Autodesk Inventor part; units mm, degrees
ref_plane "YZ Plane" through (0, 0, 0) normal (1, 0, 0) x (0, 1, 0)
ref_plane "XZ Plane" through (0, 0, 0) normal (0, 1, 0) x (-1, 0, 0)
ref_plane "XY Plane" through (0, 0, 0) normal (0, 0, 1) x (1, 0, 0)
sketch "Szkic1" plane through (0, 0, 0) normal (0, 1, 0) x (-1, 0, 0)
  line L0 (0, 0) -> (0, -40)
  line L1 (0, 0) -> (44, 0)
  line L2 (44, 0) -> (44, -40)
  line L3 (0, -40) -> (44, -40)
  dimension "d0" = 40
  dimension "d1" = 44
extrude "Wyciągnięcie proste1" add sketch "Szkic1" along normal blind 3
sketch "Szkic2" plane through (0, 3, 0) normal (0, 1, 0) x (1, 0, 0)
  line L0 (0, 0) -> (0, 40)
  line L1 (0, 40) -> (-44, 40)
  line L2 (-44, 40) -> (-44, 0)
  line L3 (-44, 0) -> (0, 0)
  line L4 (-42, 2) -> (-42, 38)
  line L5 (-42, 38) -> (-2, 38)
  line L6 (-2, 38) -> (-2, 2)
  line L7 (-2, 2) -> (-42, 2)
  line L8 (-42, 38) -> (-42, 40)
  line L9 (-2, 38) -> (-2, 40)
  line L10 (-2, 2) -> (-2, 0)
  line L11 (-42, 2) -> (-42, 0)
  dimension "d4" = 2
extrude "Wyciągnięcie proste2" add sketch "Szkic2" along normal blind 10 contours L3 L10 L6 L9 L1 L0 | L3 L2 L1 L8 L4 L11
sketch "Szkic3" plane through (0, 0, 0) normal (0, -1, 0) x (1, 0, 0)
  line L0 (0, 0) -> (0, -40)
  line L1 (-44, 0) -> (0, 0)
  line L2 (-44, -40) -> (-44, 0)
  line L3 (0, -40) -> (-44, -40)
  line L4 (0, -20) -> (5, -20)
  line L5 (-44, -20) -> (-49, -20) construction
  line L6 (-49, -20) -> (-49, -22.5)
  line L7 (-49, -20) -> (-49, -17.5)
  line L8 (5, -20) -> (5, -22.5)
  line L9 (5, -22.5) -> (5, -20)
  line L10 (5, -20) -> (5, -17.5)
  line L11 (5, -17.5) -> (0, -17.5)
  line L12 (5, -22.5) -> (0, -22.5)
  line L13 (-49, -22.5) -> (-44, -22.5)
  line L14 (-49, -17.5) -> (-44, -17.5)
  dimension "d7" = 5
  dimension "d8" = 5
  dimension "d9" = 2.5
  dimension "d10" = 2.5
  dimension "d11" = 2.5
  dimension "d12" = 2.5
extrude "Wyciągnięcie proste3" add sketch "Szkic3" against normal blind 3 contours L11 L10 L4 L0 | L4 L8 L12 L0 | L2 L13 L6 L7 L14
sketch "Szkic4" plane through (0, 3, 0) normal (0, 1, 0) x (1, 0, 0)
  line L0 (5, 17.5) -> (5, 22.5)
  line L1 (5, 22.5) -> (0, 22.5)
  line L2 (0, 17.5) -> (0, 22.5)
  line L3 (0, 17.5) -> (5, 17.5)
  line L4 (5, 17.5) -> (4, 17.5)
  line L5 (4, 17.5) -> (4, 22.5)
  line L6 (4, 22.5) -> (5, 22.5)
  line L7 (5, 22.5) -> (5, 17.5)
  line L8 (-49, 22.5) -> (-49, 17.5)
  line L9 (-49, 17.5) -> (-44, 17.5)
  line L10 (-44, 22.5) -> (-44, 17.5)
  line L11 (-44, 22.5) -> (-49, 22.5)
  line L12 (-49, 17.5) -> (-48, 17.5)
  line L13 (-48, 17.5) -> (-48, 22.5)
  line L14 (-48, 22.5) -> (-49, 22.5)
  line L15 (-49, 22.5) -> (-49, 17.5)
  point P0 (0, 0)
  dimension "d15" = 1
  dimension "d16" = 1
extrude "Wyciągnięcie proste4" add sketch "Szkic4" along normal blind 4 contours L3 L5 L1 L0 | L11 L13 L9 L8
sketch "Szkic5" plane through (4, 3, -22.5) normal (-1, 0, 0) x (0, 0, 1)
  line L0 (5, 0) -> (0, 0)
  line L1 (5, 0) -> (5, 4)
  line L2 (0, 4) -> (5, 4)
  line L3 (0, 0) -> (0, 4)
  line L4 (5, 4) -> (0, 4)
  line L5 (0, 4) -> (0, 3)
  line L6 (0, 3) -> (5, 3)
  line L7 (5, 3) -> (5, 4)
  point P0 (22.5, -3)
  dimension "d19" = 5
  dimension "d20" = 1
extrude "Wyciągnięcie proste5" add sketch "Szkic5" along normal blind 1 contours L6 L3 L2 L1
sketch "Szkic6" plane through (-48, 3, -17.5) normal (1, 0, 0) x (0, 0, -1)
  line L0 (5, 0) -> (0, 0)
  line L1 (5, 0) -> (5, 4)
  line L2 (0, 4) -> (5, 4)
  line L3 (0, 0) -> (0, 4)
  line L4 (0, 4) -> (5, 4)
  line L5 (5, 4) -> (5, 3)
  line L6 (5, 3) -> (0, 3)
  line L7 (0, 3) -> (0, 4)
  point P0 (-17.5, -3)
  point P1 (0, 3)
  point P2 (5, 3)
  dimension "d23" = 5
  dimension "d24" = 1
extrude "Wyciągnięcie proste6" add sketch "Szkic6" along normal blind 1 contours L6 L3 L2 L1
fillet "Zaokrąglenie1" radius 0.3 18 edges at (-49, 0, -20) (5, 0, -20) (5, 7, -20) (-49, 7, -20) (-44, 0, -31.25) (0, 0, -31.25) (0, 0, -8.75) (2.5, 0, -17.5) (2.5, 0, -22.5) (-44, 0, -8.75) (-46.5, 0, -17.5) (-46.5, 0, -22.5) (0, 13, -20) (-44, 13, -20) (-47, 7, -20) (3, 7, -20) (3, 6, -20) (-47, 6, -20)
sketch "Szkic8" plane through (-42, 3, 0) normal (0, 0, 1) x (1, 0, 0)
  arc A0 (-1.7, 10) -> (-2, 9.7) centre (-1.7, 9.7) ccw
  line L0 (-2, -2.7) -> (-2, 9.7)
  arc A1 (-2, -2.7) -> (-1.7, -3) centre (-1.7, -2.7) ccw
  line L1 (-1.7, -3) -> (41.7, -3)
  arc A2 (41.7, -3) -> (42, -2.7) centre (41.7, -2.7) ccw
  line L2 (42, -2.7) -> (42, 9.7)
  arc A3 (42, 9.7) -> (41.7, 10) centre (41.7, 9.7) ccw
  line L3 (40, 10) -> (41.7, 10)
  line L4 (40, 0) -> (40, 10)
  line L5 (0, 0) -> (40, 0)
  line L6 (0, 0) -> (0, 10)
  line L7 (-1.7, 10) -> (0, 10)
  point P0 (42, -3)
extrude "Wyciągnięcie proste7" add sketch "Szkic8" along normal blind 50
sketch "Szkic9" plane through (-2, 3, -40) normal (0, 0, -1) x (-1, 0, 0)
  arc A0 (42, 9.7) -> (41.7, 10) centre (41.7, 9.7) ccw
  line L0 (40, 10) -> (41.7, 10)
  line L1 (40, 0) -> (40, 10)
  line L2 (0, 0) -> (40, 0)
  line L3 (0, 0) -> (0, 10)
  line L4 (-1.7, 10) -> (0, 10)
  arc A1 (-1.7, 10) -> (-2, 9.7) centre (-1.7, 9.7) ccw
  line L5 (-2, -2.7) -> (-2, 9.7)
  arc A2 (-2, -2.7) -> (-1.7, -3) centre (-1.7, -2.7) ccw
  line L6 (-1.7, -3) -> (41.7, -3)
  arc A3 (41.7, -3) -> (42, -2.7) centre (41.7, -2.7) ccw
  line L7 (42, -2.7) -> (42, 9.7)
  point P0 (-2, -3)
extrude "Wyciągnięcie proste8" add sketch "Szkic9" along normal blind 50
sketch "Szkic10" plane through (0, 13, 0) normal (0, 1, 0) x (1, 0, 0)
  line L0 (-43.7, 90) -> (-43.7, -50)
  line L1 (-42, -50) -> (-43.7, -50)
  line L2 (-42, 90) -> (-42, -50)
  line L3 (-43.7, 90) -> (-42, 90)
  line L4 (-2, -50) -> (-2, 90)
  line L5 (-2, -50) -> (-2, 90)
  line L6 (-42, 90) -> (-2, 90)
  line L7 (-42, 90) -> (-42, -50)
  line L8 (-2, -50) -> (-42, -50)
  line L9 (-44, 22.5) -> (-48, 22.5)
  line L10 (-48, 22.5) -> (-48, 17.5)
  line L11 (-48, 17.5) -> (-44, 17.5)
  line L12 (-44, 22.5) -> (-44, 17.5)
  line L13 (-44, 22.5) -> (-48, 22.5)
  line L14 (-49, 22.5) -> (-49, 17.5)
  line L15 (-48, 22.5) -> (-48, 17.5)
  line L16 (-42, 17.5) -> (-2, 17.5)
  line L17 (-2, 17.5) -> (-2, 22.5)
  line L18 (-2, 22.5) -> (-42, 22.5)
  line L19 (-42, 22.5) -> (-42, 17.5)
  line L20 (-42, 17.5) -> (-2, 17.5)
  line L21 (-2, 17.5) -> (-2, 10.5)
  line L22 (-2, 10.5) -> (-42, 10.5)
  line L23 (-42, 10.5) -> (-42, 17.5)
  line L24 (-42, 22.5) -> (-2, 22.5)
  line L25 (-2, 22.5) -> (-2, 29.5)
  line L26 (-2, 29.5) -> (-42, 29.5)
  line L27 (-42, 29.5) -> (-42, 22.5)
  point P0 (0, 0)
  dimension "d32" = 5
  dimension "d33" = 40
  dimension "d34" = 7
  dimension "d35" = 40
  dimension "d36" = 7
extrude "Wyciągnięcie proste9" add sketch "Szkic10" against normal blind 2 contours L26 L4 L18 L2 | L2 L16 L4 L22 | L18 L4 L16 L2
properties part number "obudowa"
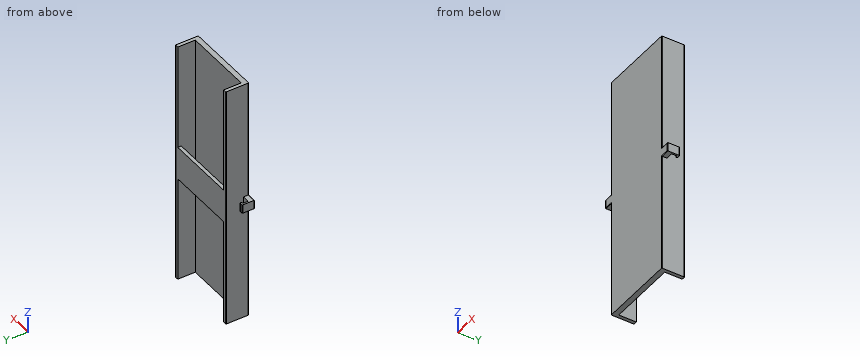
Work out the finished part from the listing and answer in its coordinate system (mm). Coordinates: 2 decimals unless noted, no trailing zeros. Write each loop counter-clockwise with the first axis right and the second up, starting at its lowest first coordinate (ties: lowest second). Pieces come first, ordered by that corner, then holes. Notation, with made-up numbers: M -20,34.5 L 26,34.5 A35 ccw 26,66.5 Z; hole C -16.5,-34 d2. An arc over 180 degrees is marked long. Answer as CSV lines item,"result". Start each with the question number.
Item 1: Section C-C on x = -20 is taken. Write down the section's boundary in (y, z), and give its area (3 significant figures).
Item 2: Consider L1, parallel to Y at x = -11, z = -17.5; L2, parallel to X at y = 8.25, z = 35; L3, parallel to Y at x = -36.5, z = -42. Determine where each line is inside the solid, lowest interval first.
Item 3: Flat-ended cylindrical pins translate along their axes: P1, Ø3, axis at y = 8.5, z = -42.5, coming from the -X side; P2, Ø5.5, axis at x = -47, y = 3, coming from the -Z side; P3, Ø5.5, axis at x = 3, y = 3, coming from the +Z side; P4, Ø21, axis at x = -12.5, z = -24, coming from the -Y side. Find the tip coordinate at first contact, or state that the pin passes through.
Item 4: Section A-A on y = 4.25 is taken. Write down the section's boundary in (x, z).
Item 5: Section D-D on z = 27.5 is taken. Write down the section's boundary in (x, y), and give its area (3 significant figures).
Item 6: Section B-B on z = -26.5 is taken. Write down the section's boundary in (x, y).
Checks:
1,outline,"M 0,-90 L 3,-90 L 3,50 L 0,50 Z; M 11,-29.5 L 13,-29.5 L 13,-10.5 L 11,-10.5 Z"
1,area,"458 mm²"
2,L1,"y = 0 to 3, 11 to 13"
2,L2,"x = -44 to -42, -2 to 0"
2,L3,"y = 0 to 3"
3,P1,"stops at x = -44"
3,P2,"stops at z = -22.5"
3,P3,"stops at z = -17.5"
3,P4,"stops at y = 0"
4,outline,"M -49,-22.5 L -48,-22.5 L -48,-17.5 L -49,-17.5 Z; M -44,-90 L -42,-90 L -42,50 L -44,50 Z; M -2,-90 L 0,-90 L 0,50 L -2,50 Z; M 4,-22.5 L 5,-22.5 L 5,-17.5 L 4,-17.5 Z"
5,outline,"M -44,0.3 A0.3 ccw -43.7,0 L -0.3,0 A0.3 ccw 0,0.3 L 0,12.7 A0.3 ccw -0.3,13 L -2,13 L -2,3 L -42,3 L -42,13 L -43.7,13 A0.3 ccw -44,12.7 Z"
5,area,"172 mm²"
6,outline,"M -44,0.3 A0.3 ccw -43.7,0 L -0.3,0 A0.3 ccw 0,0.3 L 0,12.7 A0.3 ccw -0.3,13 L -43.7,13 A0.3 ccw -44,12.7 Z; hole M -42,3 L -2,3 L -2,11 L -42,11 Z"
